Autodesk Inventor part; units mm, degrees
ref_plane "YZ Plane" through (0, 0, 0) normal (1, 0, 0) x (0, 1, 0)
ref_plane "XZ Plane" through (0, 0, 0) normal (0, 1, 0) x (-1, 0, 0)
ref_plane "XY Plane" through (0, 0, 0) normal (0, 0, 1) x (1, 0, 0)
sketch "Эскиз1" plane through (0, 0, 0) normal (0, 0, 1) x (1, 0, 0)
  circle A0 centre (-7.5, -22.95) radius 1.5
  circle A1 centre (7.5, -22.95) radius 1.5
  circle A2 centre (7.5, -6.95) radius 1.5
  circle A3 centre (-7.5, -6.95) radius 1.5
  line L0 (-281.4, 13.05) -> (10, 13.05)
  line L1 (10, 13.05) -> (10, -42.95)
  line L2 (10, -42.95) -> (-281.4, -42.95)
  line L3 (-281.4, -42.95) -> (-281.4, 13.05)
  line L4 (-281.4, 13.05) -> (10, -42.95) construction
  line L5 (10, 13.05) -> (-281.4, -42.95) construction
  line L6 (-135.7, -14.95) -> (-135.7, -42.95) construction
  circle A4 centre (-263.9, -22.95) radius 1.5
  circle A5 centre (-278.9, -22.95) radius 1.5
  circle A6 centre (-278.9, -6.95) radius 1.5
  circle A7 centre (-263.9, -6.95) radius 1.5
  point P0 (0, 0)
  dimension "d5" = 291.4
  dimension "d8" = 2.5
  dimension "d9" = 20
  dimension "d10" = 20
extrude "Выдавливание1" add sketch "Эскиз1" along normal blind 4
sketch "Эскиз4" plane through (0, 0, 0) normal (0, 0, -1) x (-1, 0, 0)
  line L0 (27.7, 31.05) -> (243.7, 31.05)
  line L1 (243.7, 31.05) -> (243.7, -4.95)
  line L2 (243.7, -4.95) -> (27.7, -4.95)
  line L3 (27.7, -4.95) -> (27.7, 31.05)
  line L4 (-10, 13.05) -> (281.4, 13.05)
  line L5 (27.7, 31.05) -> (243.7, -4.95) construction
  line L6 (243.7, 31.05) -> (27.7, -4.95) construction
  point P0 (0, 0)
  point P1 (135.7, 13.05)
  point P2 (243.7, 13.05)
  dimension "d13" = 18
  dimension "d14" = 216
extrude "Выдавливание3" cut sketch "Эскиз4" against normal blind 4
ref_plane "РабПлоскость1" through (-281.4, -14.95, 0) normal (0, -1, 0) x (1, 0, 0)
mirror "Зеркальное отражение1" about plane through (-281.4, -14.95, 0) normal (0, -1, 0) of "Выдавливание3"
sketch "Эскиз8" plane through (0, 0, 4) normal (0, 0, 1) x (1, 0, 0)
  circle A0 centre (-278.8, -36.95) radius 1.6
  line L0 (-243.7, -42.95) -> (-243.7, -24.95)
  line L1 (-281.4, -42.95) -> (-243.7, -42.95)
  circle A1 centre (-278.8, 7.05) radius 1.6
  point P0 (0, 0)
  dimension "d48" = 3.2
  dimension "d49" = 44
extrude "Выдавливание7" cut sketch "Эскиз8" against normal blind 10
ref_plane "РабПлоскость2" through (-135.7, -42.95, 0) normal (-1, 0, 0) x (0, 0, 1)
mirror "Зеркальное отражение2" about plane through (-135.7, -42.95, 0) normal (-1, 0, 0) of "Выдавливание7"
sketch "Эскиз10" plane through (0, 0, 4) normal (0, 0, 1) x (1, 0, 0)
  circle A0 centre (7.4, -36.95) radius 1.6
  circle A1 centre (-25.1, -36.95) radius 1.6
  point P0 (0, 0)
  dimension "d50" = 3.2
  dimension "d51" = 32.5
extrude "Выдавливание8" cut sketch "Эскиз10" against normal blind 10
sketch "Эскиз11" plane through (0, 0, 4) normal (0, 0, 1) x (1, 0, 0)
  circle A0 centre (-256.6, 9.05) radius 1.6
  point P0 (0, 0)
extrude "Выдавливание9" cut sketch "Эскиз11" against normal blind 10
mirror "Зеркальное отражение4" about plane through (-135.7, -42.95, 0) normal (-1, 0, 0) of "Выдавливание9"
sketch "Эскиз12" plane through (0, 0, 4) normal (0, 0, 1) x (1, 0, 0)
  circle A0 centre (-14.8, -14.95) radius 1.6
  line L0 (-243.7, -24.95) -> (-27.7, -24.95)
  circle A1 centre (-14.8, 9.05) radius 1.6
  line L1 (-14.8, -24.95) -> (-14.8, 9.05) construction
  circle A2 centre (-60.5, -14.95) radius 1.6
  circle A3 centre (-44.8, -14.95) radius 1.6
  point P0 (0, 0)
  dimension "d56" = 3.2
  dimension "d57" = 10
  dimension "d58" = 3.2
  dimension "d59" = 45.7
extrude "Выдавливание10" cut sketch "Эскиз12" against normal blind 10 contours A0 | A2 | A3
sketch "Эскиз14" plane through (-243.7, -42.95, 0) normal (1, 0, 0) x (0, 0, -1)
  line L0 (0, 56) -> (0, 38) construction
  line L1 (0, 38) -> (0, 18) construction
  line L2 (0, 18) -> (-4, 18) construction
  line L3 (-4, 0) -> (-4, 18) construction
  line L4 (0, 0) -> (-4, 0) construction
  line L5 (0, 18) -> (0, 0) construction
  line L6 (-4, 56) -> (0, 56) construction
  line L7 (-4, 38) -> (-4, 56) construction
  line L8 (-4, 38) -> (0, 38) construction
  line L9 (-4, 18) -> (-4, 38) construction
  line L10 (-4, 56) -> (0, 56)
  line L11 (0, 56) -> (0, 38)
  line L12 (0, 38) -> (-4, 38)
  line L13 (-4, 38) -> (-4, 56)
  line L14 (-4, 0) -> (-4, 18)
  line L15 (0, 18) -> (0, 0)
  line L16 (-4, 18) -> (0, 18)
  line L17 (0, 18) -> (0, 0)
  line L18 (0, 0) -> (-4, 0)
  line L19 (-4, 0) -> (-4, 18)
  point P0 (0, 42.95)
  point P1 (0, 18)
extrude "Выдавливание12" cut sketch "Эскиз14" against normal blind 9.5
properties part number "центр_рейка" material "Древесина (береза)"
Here's how the part is built. I have some questions about the finished solid (model axes, mm). Round coordinates to 2 decimals unless told otherwise and drop trailing zeros. Write each loop counter-clockwise with the first axis right and the second up, starting at its lowest first coordinate (ties: lowest second). Pieces come first, ordered by that corner, then holes.
1. Suppose I cut it at B-B (y = -30). List the corners of the cut face in (x, z) for me.
2. Suppose I cut it at A-A (z = 0.75). State how many separate pieces and enclosed holes the cut face has, and give its area (3 significant figures).
3. Suppose I cut it at C-C (x = -213). List the corners of the cut face in (y, z) for me.
4. Will these pins go through, and if not, where does the flat tip stop? pin 1 Ø1.2 at (x, z) = (-106, 2.5) entering from +Y; pin 2 Ø1.9 at (x, y) = (-14.8, -14.95) entering from +Z.
5. I need wall thicknesses on L1, parallel to Y at x = -14.8, z = 1.9; L2, parallel to Y at x = -278.9, z = 2.2; L3, parallel to Y at x = -263.9, z = 3.15. Which ranges of each line are inside material? Lowest first, please.
Answer sheet:
1. outline: (-281.4, 0) - (-253.2, 0) - (-253.2, 4) - (-281.4, 4) - close; (-27.7, 0) - (10, 0) - (10, 4) - (-27.7, 4) - close
2. separate pieces: 1
2. enclosed holes: 18
2. area: 8,060 mm2
3. outline: (-24.95, 0) - (-4.95, 0) - (-4.95, 4) - (-24.95, 4) - close
4. pin 1: stops at y = -4.95
4. pin 2: passes through
5. L1: y = -42.95 to -16.55, -13.35 to 7.45, 10.65 to 13.05
5. L2: y = -42.95 to -38.55, -35.35 to -24.45, -21.45 to -8.45, -5.45 to 5.45, 8.65 to 13.05
5. L3: y = -42.95 to -24.45, -21.45 to -8.45, -5.45 to 13.05
